Input: part model. Units: mm. Frame: model coordinates. Give positions to 0.01 mm unless a question says otherwise; leave off trailing zeros. Order: outer loops, then holes, each group sorted by start corner. A loop starts at its lowest first (then second) coordinate and runs counter-clockwise, first axis right, second up. Notation, with made-up numbers: (64, -20.75) - (71, -20.75) arc R19 ccw to (71, -5.75) - close; hole circle Ø6 at (13, -27). An arc over 180 degrees is marked (long way). Answer in a Markdown table with one row per item. Add a question column.
from build123d import *

# Parameters (mm, degrees)
BASPROSKE_W           = 20
BASPROSKE_H           = 9
TOOTHCUT_DEPTH        = 24.706539182
TEETHCUTS_COUNT       = 10
TEETHCUTS_ANGLE       = 324
BORSKE_R              = 2.5
BORE_DEPTH            = 50.0000508
IZIM1_R               = 3
KES_EKSTR_ZYON1_DEPTH = 26


with BuildPart() as part:
    # BasProSke → Base-Revolve (revolve)
    with BuildSketch(Plane(origin=(0, 0, 0), x_dir=(1, 0, 0), z_dir=(0, 1, 0)), mode=Mode.PRIVATE) as base_revolve_sk:
        with Locations((10, 4.5)):
            Rectangle(BASPROSKE_W, BASPROSKE_H)
    revolve(base_revolve_sk.sketch.rotate(Axis((-10, 0, 0), (1, 0, 0)), 180), axis=Axis((-10, 0, 0), (1, 0, 0)))

    # TooCutSke → ToothCut (cut, through all)
    with BuildSketch(Plane(origin=(0, 0, 0), x_dir=(0, 0, -1), z_dir=(1, 0, 0))):
        with BuildLine():
            ThreePointArc((0.883878355, 5.554109745), (0, 5.624), (-0.883878355, 5.554109745))
            ThreePointArc((-0.883878355, 5.554109745), (-1.258245767, 7.379188248), (-2.637816971, 8.631324741))
            ThreePointArc((-2.637816971, 8.631324741), (0, 9.0254), (2.637816971, 8.631324741))
            ThreePointArc((2.637816971, 8.631324741), (1.258245767, 7.379188248), (0.883878355, 5.554109745))
        make_face()
    toothcut = extrude(amount=TOOTHCUT_DEPTH, mode=Mode.SUBTRACT)

    # TeethCuts: ToothCut ×10 about axis
    teethcuts_axis = Axis((-10, 0, 0), (1, 0, 0))
    for i in range(1, TEETHCUTS_COUNT):
        add(toothcut.rotate(teethcuts_axis, i * TEETHCUTS_ANGLE / (TEETHCUTS_COUNT - 1)), mode=Mode.SUBTRACT)

    # BorSke → Bore (cut, symmetric)
    with BuildSketch(Plane(origin=(0, 0, 0), x_dir=(0, 0, -1), z_dir=(1, 0, 0))):
        with Locations(Location((0, 0, 0), (0, 0, 180))):
            Circle(BORSKE_R)
    extrude(amount=BORE_DEPTH, both=True, mode=Mode.SUBTRACT)

    # Çizim1 → Kes-Ekstrüzyon1 (cut)
    with BuildSketch(Plane(origin=(20, 0, 0), x_dir=(0, 0, -1), z_dir=(1, 0, 0))):
        Circle(IZIM1_R)
    extrude(amount=-KES_EKSTR_ZYON1_DEPTH, mode=Mode.SUBTRACT)


solid = part.part
Q1. Section B-B, the plane z = -4.5. Return loops of the section in (x, y), then the cut area to 3 significant figures.
Q2. Line query: probe 1 along Y at (x, z) = (15, 0); probe 2 along Z at (x, y) = (14.25, -6.5); probe 3 along Z at (x, y) = (16.75, 7). Output: solid intervals per line, ascending.
Q3. Pull-direction query (Z, two-part tool) for faces 1 (the flat face through (20, 4, 0)), 2 (the cylindrical face through (9.86, -1.092, -7.362)); classes: +Z half, -Z half, draft (parallel to the pull), parting line (faces both ways), or undercut.
Q4. Contact query for flat-ended pins moving along their axis: P1, Ø1, axis at x = 3, z = -6.5, coming from the -Y side; P2, Ø1.5, axis at y = 6.5, z = -5, coming from the +X side; P3, Ø1, axis at x = 3, z = 2, coming from the +Y side. Output: stop coordinate, or through.
Q5. Section A-A, the plane z = 0. Return loops of the section in (x, y), then the cut area to 3 significant figures.
Computed:
| question | item | result |
|---|---|---|
| 1 | outline | (0, -4.65) - (20, -4.65) - (20, 4.65) - (0, 4.65) - close |
| 1 | area | 186 mm^2 |
| 2 | probe 1 | y = -5.62 to -3, 3 to 5.62 |
| 2 | probe 2 | z = -3.29 to -0.93, 0.93 to 3.29 |
| 2 | probe 3 | z = -3.34 to -1.08, 1.08 to 3.34 |
| 3 | face 1 | draft |
| 3 | face 2 | undercut |
| 4 | P1 | stops at y = -5.5 |
| 4 | P2 | passes through |
| 4 | P3 | stops at y = 8.57 |
| 5 | outline | (0, -5.62) - (20, -5.62) - (20, -3) - (0, -3) - close; (0, 3) - (20, 3) - (20, 5.62) - (0, 5.62) - close |
| 5 | area | 105 mm^2 |
